Autodesk Fusion 360 part; units mm, degrees
sketch "Sketch1" plane through (0, 0, 0) normal (0, 0, 1) x (1, 0, 0)
  line L0 (-15.5, 12.25) -> (15.5, 12.25)
  line L1 (15.5, 12.25) -> (15.5, -12.25)
  line L2 (15.5, -12.25) -> (-15.5, -12.25)
  line L3 (-15.5, -12.25) -> (-15.5, 12.25)
  line L4 (-15.5, 12.25) -> (15.5, -12.25) construction
  line L5 (15.5, 12.25) -> (-15.5, -12.25) construction
  dimension "d1" = 31
  dimension "d2" = 24.5
extrude "Extrude1" add sketch "Sketch1" along normal blind 5.5
shell "Shell1" thickness 1.8 removed faces 1 at (-5.1667, 4.0833, 5.5)
sketch "Sketch2" plane through (0, 0, 5.5) normal (0, 0, 1) x (-1, 0, 0)
  line L0 (13.7, 10.45) -> (13.7, -10.45)
  line L1 (13.7, -10.45) -> (-13.7, -10.45)
  line L2 (-13.7, -10.45) -> (-13.7, 10.45)
  line L3 (-13.7, 10.45) -> (13.7, 10.45)
  line L4 (15.5, 12.25) -> (-15.5, 12.25)
  line L5 (-15.5, 12.25) -> (-15.5, -12.25)
  line L6 (-15.5, -12.25) -> (15.5, -12.25)
  line L7 (15.5, -12.25) -> (15.5, 12.25)
  circle A0 centre (14.4, -11.2) radius 0.84
  line L8 (0, 0) -> (0, -2)
  line L9 (0, 0) -> (4, 0)
  circle A1 centre (-14.4, -11.2) radius 0.84
  circle A2 centre (-14.4, 11.2) radius 0.84
  circle A3 centre (14.4, 11.2) radius 0.84
  dimension "d6" = 1.68
  dimension "d7" = 11.2
  dimension "d8" = 14.4
extrude "Extrude2" add sketch "Sketch2" along normal blind 4 contours A0 | A1 | A2 | A3
fillet "Fillet1" radius 1 1 edges at (15.5, -12.25, 2.75)
fillet "Fillet1" radius 1 1 edges at (15.5, 12.25, 2.75)
fillet "Fillet1" radius 1 1 edges at (-15.5, 12.25, 2.75)
fillet "Fillet1" radius 1 1 edges at (-15.5, -12.25, 2.75)
sketch "Sketch3" plane through (-15.5, 0, 0) normal (-1, 0, 0) x (0, -1, 0)
  line L0 (11.25, 0) -> (11.25, 5.5)
  line L1 (11.25, 5.5) -> (-11.25, 5.5)
  line L2 (-11.25, 5.5) -> (-11.25, 0)
  line L3 (-11.25, 0) -> (11.25, 0)
  line L4 (0, 0) -> (0, 1.96)
  line L5 (0, 1.96) -> (0, 3.46)
  line L6 (-3.4, 1.96) -> (3.4, 1.96)
  line L7 (4.4, 2.96) -> (4.4, 3.96)
  line L8 (3.4, 4.96) -> (-3.4, 4.96)
  line L9 (-4.4, 3.96) -> (-4.4, 2.96)
  line L10 (-4.4, 1.96) -> (4.4, 4.96) construction
  line L11 (4.4, 1.96) -> (-4.4, 4.96) construction
  arc A0 (-3.4, 4.96) -> (-4.4, 3.96) centre (-3.4, 3.96) ccw
  arc A1 (-4.4, 2.96) -> (-3.4, 1.96) centre (-3.4, 2.96) ccw
  arc A2 (3.4, 1.96) -> (4.4, 2.96) centre (3.4, 2.96) ccw
  arc A3 (4.4, 3.96) -> (3.4, 4.96) centre (3.4, 3.96) ccw
  point P0 (0, 3.46)
  dimension "d19" = 1.96
  dimension "d20" = 1.5
  dimension "d21" = 3
  dimension "d22" = 8.8
  dimension "d23" = 1
extrude "Extrude3" cut sketch "Sketch3" against normal blind 6 contours L6 L7 L8 L9 A0 A1 A2 A3
fillet "Fillet2" radius 0.75 8 edges at (-15.2071, -11.9571, 0) (-15.5, 0, 0) (-15.2071, 11.9571, 0) (0, 12.25, 0) (15.2071, 11.9571, 0) (15.5, 0, 0) (15.2071, -11.9571, 0) (0, -12.25, 0)
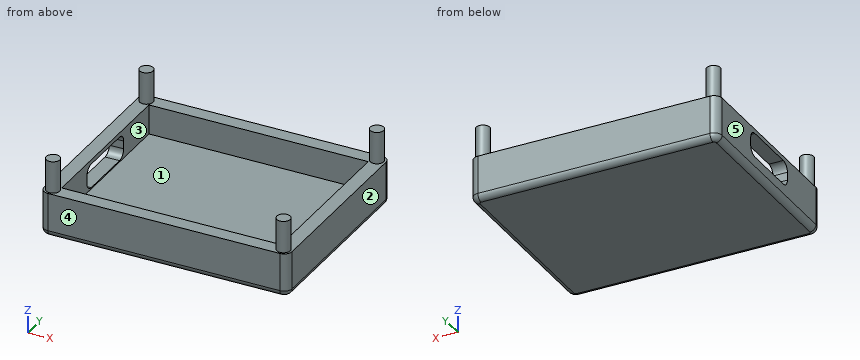
Here's how the part is built. I have some questions about the finished solid (model axes, mm). Face numbers are marked on the shaded views. A direction names the side the tool comes from. Round coordinates to 2 decimals unless told otherwise and drop trailing zeros. Loops run counter-clockwise (first coordinate to the right, second up) from the corner with the lowest first, then second, coordinate; pieces in that order, holes last. Notation, with made-up numbers: M 76.25,86 L 93.25,86 A21 cw 93.25,123 Z; hole C -14,18.5 d10. An arc over 180 degrees is marked long. Write each question's results on one line, items separated by ' | '. Start each with the question number.
(1) Will these pins go through, and if not, where does the flat tip stop? P1, Ø2, axis at x = -5, y = -2.5, coming from the +Z side; P2, Ø1.1, axis at y = 1, z = 3, coming from the -X side; P3, Ø1.5, axis at y = -9.5, z = 8, coming from the -X side; P4, Ø0.5, axis at x = -15, y = 1, coming from the +Z side.
(2) If I drill on probe 1 along Y at (x, z) = (9.5, 4); probe 2 along X at (y, z) = (-10, 5.25); probe 3 along Z at (x, y) = (-2.5, 11.5), over which ranges is the centre line in solid material (lowest first)? Write a range as from..to.
(3) I want a section at D-D (z = 6.25). Please give me the cut outline in (x, y), then the cut area to 3 significant figures.
(4) On a 3-axis mill with a long thin cutter (end or side, diameter ignored), from which of +Z, -Z, +X, -X, +Y, -Y can I reach the whole of each face in a straight line? I mean the marked faces 1 and 2. Say none if no direction works.
(5) I want a section at A-A (x = 8). Please give me the cut outline in (y, z).
(6) Thinking about a two-plate mould opening in X: for the marked faces 3, 4 and 5, which applies, pulls with the +X half, pulls with the -X half, needs draft (parallel to the pull), parting line crosses it, or undercut?
(7) I want a section at B-B (y = 8). Please give me the cut outline in (x, z).
(8) I want a section at C-C (y = 2.25). Please give me the cut outline in (x, z), then the cut area to 3 significant figures.
Solved:
1) P1: stops at z = 1.8 | P2: stops at x = 13.7 | P3: passes through | P4: stops at z = 5.5
2) probe 1: y = -12.25..-10.45, 10.45..12.25 | probe 2: x = -15.5..-13.7, 13.7..15.5 | probe 3: z = 0..5.5
3) outline: C -14.4,-11.2 d1.68; C -14.4,11.2 d1.68; C 14.4,-11.2 d1.68; C 14.4,11.2 d1.68 | area: 8.87 mm²
4) face 1: +Z | face 2: +Z, -Z, +X, +Y, -Y
5) outline: M -12.25,0.75 A0.75 ccw -11.5,0 L 11.5,0 A0.75 ccw 12.25,0.75 L 12.25,5.5 L 10.45,5.5 L 10.45,1.8 L -10.45,1.8 L -10.45,5.5 L -12.25,5.5 Z
6) face 3: undercut | face 4: needs draft | face 5: pulls with the -X half
7) outline: M -15.5,0.75 A0.75 ccw -14.75,0 L 14.75,0 A0.75 ccw 15.5,0.75 L 15.5,5.5 L 13.7,5.5 L 13.7,1.8 L -13.7,1.8 L -13.7,5.5 L -15.5,5.5 Z
8) outline: M -15.5,0.75 A0.75 ccw -14.75,0 L 14.75,0 A0.75 ccw 15.5,0.75 L 15.5,5.5 L 13.7,5.5 L 13.7,1.8 L -13.7,1.8 L -13.7,1.96 L -15.5,1.96 Z; M -15.5,4.96 L -13.7,4.96 L -13.7,5.5 L -15.5,5.5 Z | area: 63.5 mm²
